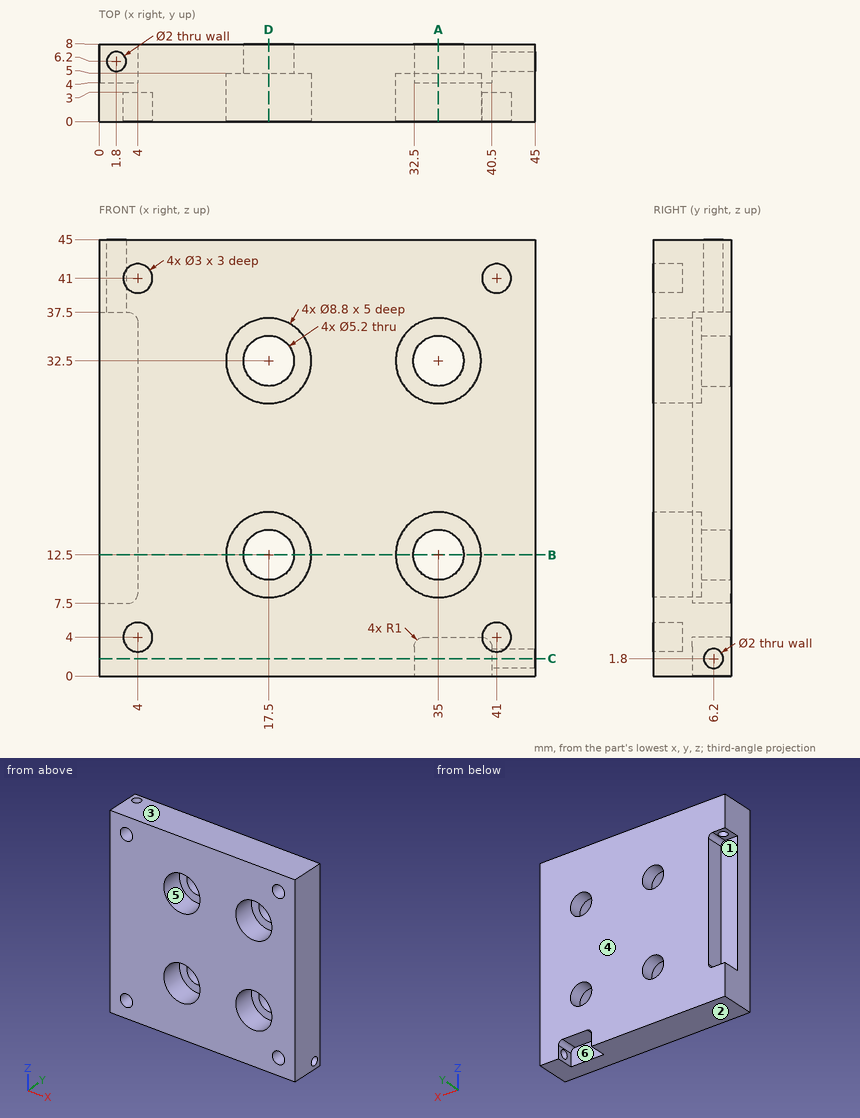
For this review, use the dimensioned drawing (mm, ordinates from the lowest corner) and the shaded views. A direction names the side the tool comes from. Coordinates: 2 decimals unless noted, no trailing zeros. Loops run counter-clockwise (first coordinate to the right, second up) from the corner with the lowest first, then second, coordinate; pieces in that order, holes last. Notation, with made-up numbers: (5, 3) -> (30, 3) arc R31 cw to (30, 35) -> close; hole circle Ø4 at (20.5, -15.75). An arc over 180 degrees is marked (long way). Use a Markdown table: item, result. Add a question column.
1. To check wall thickness, follow line 1 (Z direction, x = 17.5, y = 6.55); line 2 (Z direction, x = 41, y = 1.85); line 3 (X direction, y = 2.8, z = 32.5). State the ranges of each line that lie inside material, in increasing order.
2. Add section D-D on x = 17.5. Write out the cut boundary in (y, z).
3. Add section B-B on z = 12.5. Write out the cut boundary in (x, y), plus the area to 3 significant figures.
4. Draft analysis for pull direction Z (two halves, no side actions). For the marked faces 1, 2 and 3, state which applies: pulls with the +Z half, pulls with the -Z half, needs draft (parallel to the pull), parting line crosses it, or undercut.
5. Add section C-C on z = 1.8. Write out the cut boundary in (x, y), plus the area to 3 significant figures.
6. Machinability: for the marked faces 4, 5 and 6, which of the approach directions +Z, -Z, +X, -X, +Y, -Y give a long, thin tool a straight path to every point of the face, cutting with its end or side? Answer none if there is none.
7. Add section A-A on x = 35. Write out the cut boundary in (y, z), plus the area to 3 significant figures.
8. Clearance check with flat-ended pins moving along their axes: pin 1 Ø2 at (x, y) = (36, 5.5) entering from -Z; pin 2 Ø4.5 at (x, z) = (18, 32) entering from -Y; pin 3 Ø1.5 at (x, z) = (4, 4) entering from -Y. State where each tip first meets the part, or that it passes through.
Returned:
| question | item | result |
|---|---|---|
| 1 | line 1 | z = 0 to 9.9, 15.1 to 29.9, 35.1 to 45 |
| 1 | line 2 | z = 0 to 2.5, 5.5 to 39.5, 42.5 to 45 |
| 1 | line 3 | x = 0 to 13.1, 21.9 to 30.6, 39.4 to 45 |
| 2 | outline | (0, 0) -> (8, 0) -> (8, 9.9) -> (5, 9.9) -> (5, 8.1) -> (0, 8.1) -> close; (0, 16.9) -> (5, 16.9) -> (5, 15.1) -> (8, 15.1) -> (8, 29.9) -> (5, 29.9) -> (5, 28.1) -> (0, 28.1) -> close; (0, 36.9) -> (5, 36.9) -> (5, 35.1) -> (8, 35.1) -> (8, 45) -> (0, 45) -> close |
| 3 | outline | (0, 0) -> (13.1, 0) -> (13.1, 5) -> (14.9, 5) -> (14.9, 8) -> (4, 8) -> (4, 4) -> (0, 4) -> close; (20.1, 5) -> (21.9, 5) -> (21.9, 0) -> (30.6, 0) -> (30.6, 5) -> (32.4, 5) -> (32.4, 8) -> (20.1, 8) -> close; (37.6, 5) -> (39.4, 5) -> (39.4, 0) -> (45, 0) -> (45, 8) -> (37.6, 8) -> close |
| 3 | area | 225 mm² |
| 4 | face 1 | undercut |
| 4 | face 2 | pulls with the -Z half |
| 4 | face 3 | pulls with the +Z half |
| 5 | outline | (0, 0) -> (45, 0) -> (45, 5.2) -> (40.5, 5.2) -> (40.5, 4) -> (32.5, 4) -> (32.5, 8) -> (0, 8) -> close; (40.5, 7.2) -> (45, 7.2) -> (45, 8) -> (40.5, 8) -> close |
| 5 | area | 319 mm² |
| 6 | face 4 | +Z, -Z, +X, -X, +Y |
| 6 | face 5 | -Y |
| 6 | face 6 | -Z, +Y |
| 7 | outline | (0, 0) -> (4, 0) -> (4, 4) -> (8, 4) -> (8, 9.9) -> (5, 9.9) -> (5, 8.1) -> (0, 8.1) -> close; (0, 16.9) -> (5, 16.9) -> (5, 15.1) -> (8, 15.1) -> (8, 29.9) -> (5, 29.9) -> (5, 28.1) -> (0, 28.1) -> close; (0, 36.9) -> (5, 36.9) -> (5, 35.1) -> (8, 35.1) -> (8, 45) -> (0, 45) -> close |
| 7 | area | 225 mm² |
| 8 | pin 1 | stops at z = 4 |
| 8 | pin 2 | stops at y = 5 |
| 8 | pin 3 | stops at y = 3 |
